For this review, use the dimensioned drawing (mm, ordinates from the lowest corner) and the shaded views. A direction names the side the tool comes from. Coordinates: 2 decimals unless noted, no trailing zeros. Write each loop counter-clockwise with the first axis right and the second up, starting at its lowest first coordinate (ties: lowest second). Pieces come first, ordered by that corner, then holes. Notation, with made-up numbers: M 17.25,10.25 L 68.25,10.25 A35 cw 68.25,48.25 Z; hole C -21,67.25 d11. An arc over 180 degrees is marked long. One line per question, with ' | ' between items.
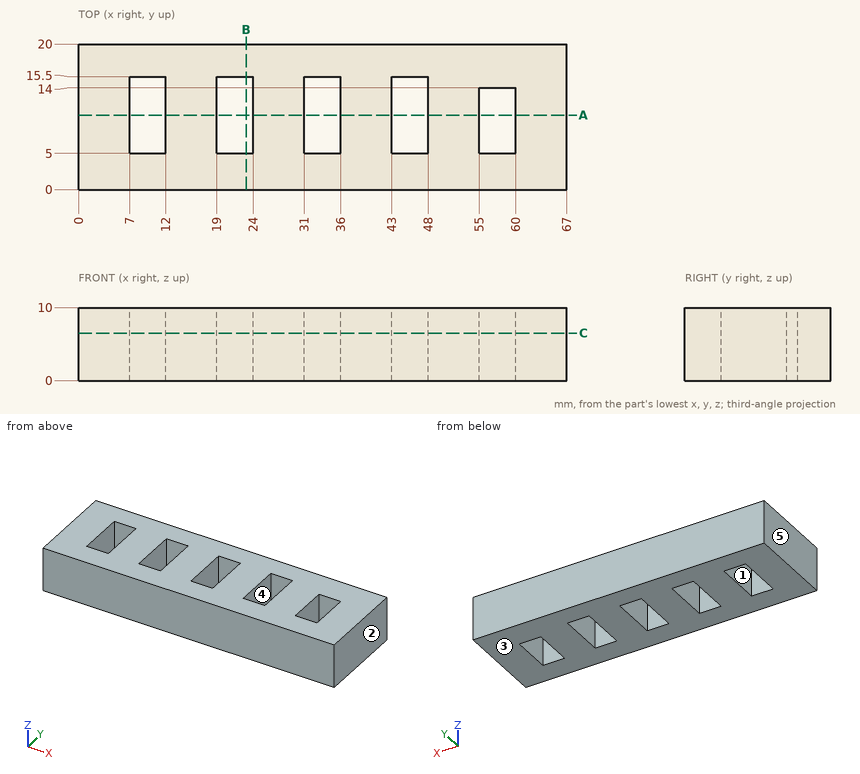
1) To check wall thickness, follow line 1 along X through (y, z) = (12.75, 8.75); line 2 along Y through (x, z) = (20, 8.25); line 3 along Y through (x, z) = (57, 3). State the ranges of each line that lie inside material, in increasing order. Write a range as [from, to].
Responses:
line 1: [0, 7], [12, 19], [24, 31], [36, 43], [48, 55], [60, 67] | line 2: [0, 5], [15.5, 20] | line 3: [0, 5], [14, 20]
2) Machinability: for the marked faces 1 and 2, which of the approach directions +Z, -Z, +X, -X, +Y, -Y give a long, thin tool a straight path to every point of the face, cutting with its end or side? Answer none if there is none.
Responses:
face 1: +Z, -Z | face 2: +Z, -Z, +X, +Y, -Y
3) We need section A-A on y = 10.25. State the section outline as (x, z) points, then the cut area to 3 significant figures.
Responses:
outline: M 0,0 L 7,0 L 7,10 L 0,10 Z; M 12,0 L 19,0 L 19,10 L 12,10 Z; M 24,0 L 31,0 L 31,10 L 24,10 Z; M 36,0 L 43,0 L 43,10 L 36,10 Z; M 48,0 L 55,0 L 55,10 L 48,10 Z; M 60,0 L 67,0 L 67,10 L 60,10 Z | area: 420 mm^2
4) We need section C-C on z = 6.5. State the section outline as (x, y) points, then the cut area to 4 significant figures.
Responses:
outline: M 0,0 L 67,0 L 67,20 L 0,20 Z; hole M 7,5 L 12,5 L 12,15.5 L 7,15.5 Z; hole M 19,5 L 24,5 L 24,15.5 L 19,15.5 Z; hole M 31,5 L 36,5 L 36,15.5 L 31,15.5 Z; hole M 43,5 L 48,5 L 48,15.5 L 43,15.5 Z; hole M 55,5 L 60,5 L 60,14 L 55,14 Z | area: 1,085 mm^2
5) We need section B-B on x = 23. State the section outline as (y, z) points, then the cut area to 3 significant figures.
Responses:
outline: M 0,0 L 5,0 L 5,10 L 0,10 Z; M 15.5,0 L 20,0 L 20,10 L 15.5,10 Z | area: 95.0 mm^2
6) The part is to be moulded in two halves that separate along X. For the marked faces 3, 4 and 5, say which applies: +X half, -X half, draft (parallel to the pull), parting line (faces both ways), or undercut.
Responses:
face 3: draft | face 4: undercut | face 5: -X half
